Autodesk Inventor part; units mm, degrees
ref_plane "YZ Plane" through (0, 0, 0) normal (1, 0, 0) x (0, 1, 0)
ref_plane "XZ Plane" through (0, 0, 0) normal (0, 1, 0) x (-1, 0, 0)
ref_plane "XY Plane" through (0, 0, 0) normal (0, 0, 1) x (1, 0, 0)
sketch "Sketch1" plane through (0, 0, 0) normal (0, 1, 0) x (-1, 0, 0)
  line L0 (95, 92.5) -> (-95, 92.5)
  line L1 (-95, 92.5) -> (-95, -92.5)
  line L2 (-95, -92.5) -> (95, -92.5)
  line L3 (95, -92.5) -> (95, 92.5)
  point P0 (0, 0)
  dimension "d0" = 190
  dimension "d1" = 185
  dimension "d2" = 95
  dimension "d3" = 92.5
extrude "Extrusion1" add sketch "Sketch1" along normal blind 5
sketch "Sketch2" plane through (0, 0, 0) normal (0, -1, 0) x (1, 0, 0)
  line L0 (90, 87.5) -> (-90, 87.5)
  line L1 (-90, 87.5) -> (-90, -87.5)
  line L2 (-90, -87.5) -> (90, -87.5)
  line L3 (90, -87.5) -> (90, 87.5)
  line L4 (-95, 92.5) -> (95, 92.5)
  line L5 (-95, -92.5) -> (-95, 92.5)
  line L6 (95, -92.5) -> (-95, -92.5)
  line L7 (95, 92.5) -> (95, -92.5)
  line L8 (95, 92.5) -> (-95, 92.5)
  line L9 (-95, 92.5) -> (-95, -92.5)
  line L10 (-95, -92.5) -> (95, -92.5)
  line L11 (95, -92.5) -> (95, 92.5)
  point P0 (0, 0)
  dimension "d109" = 5
  dimension "d110" = 5
  dimension "d111" = 5
  dimension "d112" = 5
extrude "Extrusion2" add sketch "Sketch2" along normal blind 15
sketch "Sketch3" plane through (0, 5, 0) normal (0, 1, 0) x (1, 0, 0)
  circle A0 centre (-50, 0) radius 15.5
  point P0 (0, 0)
  dimension "d12" = 31
  dimension "d13" = 50
extrude "Extrusion3" cut sketch "Sketch3" against normal through all
sketch "Sketch4" plane through (0, 5, 0) normal (0, 1, 0) x (1, 0, 0)
  circle A0 centre (-50, 0) radius 15.5
  line L0 (-95, -92.5) -> (95, -92.5)
  line L1 (95, -92.5) -> (95, 92.5)
  line L2 (95, 92.5) -> (-95, 92.5)
  line L3 (-95, 92.5) -> (-95, -92.5)
  circle A1 centre (-77.5, -75) radius 7.5
  circle A2 centre (-77.5, 75) radius 7.5
  circle A3 centre (77.5, -75) radius 7.5
  circle A4 centre (77.5, 75) radius 7.5
  circle A5 centre (-77.5, -75) radius 8.5
  circle A6 centre (-77.5, 75) radius 8.5
  circle A7 centre (77.5, 75) radius 8.5
  circle A8 centre (77.5, -75) radius 8.5
  point P0 (0, 0)
  dimension "d16" = 15
  dimension "d17" = 17.5
  dimension "d18" = 17.5
  dimension "d19" = 15
  dimension "d20" = 15
  dimension "d21" = 15
  dimension "d22" = 17.5
  dimension "d23" = 17.5
  dimension "d24" = 17.5
  dimension "d25" = 17.5
  dimension "d26" = 17.5
  dimension "d27" = 17.5
  dimension "d28" = 17
  dimension "d29" = 17
  dimension "d30" = 17
  dimension "d31" = 17
  dimension "d34" = 75
  dimension "d35" = 77.5
extrude "Extrusion4" [suppressed]
sketch "Sketch8" plane through (0, 5, 0) normal (0, 1, 0) x (1, 0, 0)
  circle A0 centre (-50, 0) radius 15.5
  line L0 (-95, -92.5) -> (95, -92.5)
  line L1 (95, -92.5) -> (95, 92.5)
  line L2 (95, 92.5) -> (-95, 92.5)
  line L3 (-95, 92.5) -> (-95, -92.5)
  line L4 (-50, 13.5) -> (-50, -13.5)
  line L5 (-50, 13.5) -> (-95, 13.5)
  line L6 (-50, -13.5) -> (-95, -13.5)
  line L7 (-95, -13.5) -> (-95, 13.5)
  point P0 (0, 0)
  dimension "d51" = 27
  dimension "d52" = 13.5
  dimension "d62" = 31
extrude "Extrusion8" [suppressed]
sketch "Sketch10" plane through (-115, 5, -13.5) normal (0, 0, 1) x (1, 0, 0)
  line L0 (5, -20) -> (0, -20)
  line L1 (5, -5) -> (5, -20)
  line L2 (65, -5) -> (5, -5)
  line L3 (65, 0) -> (65, -5)
  line L4 (0, 0) -> (65, 0)
  line L5 (0, -20) -> (0, 0)
  line L6 (5, -17.5) -> (2.5, -17.5)
  line L7 (2.5, -17.5) -> (2.5, -2.5)
  line L8 (2.5, -2.5) -> (5, -2.5)
  line L9 (5, -2.5) -> (5, -17.5)
  line L10 (62.5, -5) -> (2.5, -5)
  line L11 (2.5, -5) -> (2.5, -2.5)
  line L12 (2.5, -2.5) -> (62.5, -2.5)
  line L13 (62.5, -2.5) -> (62.5, -5)
  point P0 (115, -5)
  dimension "d64" = 2.5
  dimension "d65" = 15
  dimension "d67" = 2.5
  dimension "d68" = 2.5
  dimension "d71" = 2.5
  dimension "d72" = 0
extrude "Extrusion10" [suppressed]
mirror "Mirror3" [suppressed]
sketch "Sketch12" plane through (0, 5, 0) normal (0, 1, 0) x (1, 0, 0)
  line L0 (-114.5, 13.5) -> (-109.5, 13.5)
  line L1 (-109.5, 13.5) -> (-109.5, 87.5)
  line L2 (-109.5, 87.5) -> (109.5, 87.5)
  line L3 (109.5, 87.5) -> (109.5, -87.5)
  line L4 (109.5, -87.5) -> (-109.5, -87.5)
  line L5 (-109.5, -87.5) -> (-109.5, -13.5)
  line L6 (-109.5, -13.5) -> (-114.5, -13.5)
  line L7 (-114.5, -13.5) -> (-114.5, -92.5)
  line L8 (-114.5, -92.5) -> (114.5, -92.5)
  line L9 (114.5, -92.5) -> (114.5, 92.5)
  line L10 (114.5, 92.5) -> (-114.5, 92.5)
  line L11 (-114.5, 92.5) -> (-114.5, 13.5)
  line L12 (-89.25, -92.5) -> (-79.25, -92.5)
  line L13 (-79.25, -92.5) -> (-79.25, -90)
  line L14 (-79.25, -90) -> (-89.25, -90)
  line L15 (-89.25, -90) -> (-89.25, -92.5)
  line L16 (79.25, -92.5) -> (89.25, -92.5)
  line L17 (89.25, -92.5) -> (89.25, -90)
  line L18 (89.25, -90) -> (79.25, -90)
  line L19 (79.25, -90) -> (79.25, -92.5)
  line L20 (-89.25, 92.5) -> (-79.25, 92.5)
  line L21 (-79.25, 92.5) -> (-79.25, 90)
  line L22 (-79.25, 90) -> (-89.25, 90)
  line L23 (-89.25, 90) -> (-89.25, 92.5)
  line L24 (79.25, 92.5) -> (89.25, 92.5)
  line L25 (89.25, 92.5) -> (89.25, 90)
  line L26 (89.25, 90) -> (79.25, 90)
  line L27 (79.25, 90) -> (79.25, 92.5)
  point P0 (0, 0)
  point P1 (0, 0)
  dimension "d87" = 10
  dimension "d88" = 2.5
  dimension "d89" = 20.25
  dimension "d90" = 10
  dimension "d91" = 2.5
  dimension "d92" = 20.25
  dimension "d93" = 2.5
  dimension "d94" = 10
  dimension "d95" = 20.25
  dimension "d96" = 2.5
  dimension "d97" = 10
  dimension "d98" = 20.25
  dimension "d113" = 5
  dimension "d114" = 5
  dimension "d115" = 5
  dimension "d116" = 5
  dimension "d117" = 5
  dimension "d118" = 229
  dimension "d119" = 229
  dimension "d120" = 158.5
  dimension "d121" = 79.25
  dimension "d122" = 79.25
extrude "Extrusion12" cut sketch "Sketch12" against normal blind 6 contours L10 L21 L22 L23 | L10 L25 L26 L27 | L8 L19 L18 L17 | L15 L14 L13 L8
sketch "Sketch13" plane through (0, -15, 0) normal (0, -1, 0) x (1, 0, 0)
  line L0 (-90, -87.5) -> (-90, 87.5)
  line L1 (-90, 87.5) -> (90, 87.5)
  line L2 (90, 87.5) -> (90, -87.5)
  line L3 (90, -87.5) -> (-90, -87.5)
  line L4 (-95, 92.5) -> (-95, -92.5)
  line L5 (-95, -92.5) -> (95, -92.5)
  line L6 (95, -92.5) -> (95, 92.5)
  line L7 (95, 92.5) -> (-95, 92.5)
  line L8 (112.75, -90.25) -> (-112.75, -90.25)
  line L9 (-112.75, -90.25) -> (-112.75, 90.25)
  line L10 (-112.75, 90.25) -> (112.75, 90.25)
  line L11 (112.75, 90.25) -> (112.75, -90.25)
  point P0 (0, 0)
  dimension "d101" = 185
  dimension "d102" = 180.5
  dimension "d104" = 225.5
  dimension "d105" = 112.75
  dimension "d106" = 90.25
extrude "Extrusion13" [suppressed]
equation "\"d110\" = d109"
equation "\"d111\" = d109"
equation "\"d112\" = d109"
equation "\"d18\" = d17"
equation "\"d19\" = d16"
equation "\"d20\" = d16"
equation "\"d21\" = d16"
equation "\"d22\" = d17"
equation "\"d23\" = d22"
equation "\"d24\" = d17"
equation "\"d25\" = d24"
equation "\"d26\" = d17"
equation "\"d27\" = d26"
equation "\"d29\" = d28"
equation "\"d30\" = d28"
equation "\"d31\" = d28"
equation "\"d52\" = 0.5 * d51"
equation "\"d90\" = d87"
equation "\"d91\" = d88"
equation "\"d92\" = d89"
equation "\"d93\" = d88"
equation "\"d94\" = d87"
equation "\"d95\" = d89"
equation "\"d96\" = d88"
equation "\"d97\" = d87"
equation "\"d98\" = d89"
properties part number "Bottom Roof"
Geometry: final body of the model. Coordinates: model frame, mm. A direction names the side the tool comes from. Coordinates: 2 decimals unless noted, no trailing zeros. Order: outer loops, then holes, each group sorted by start corner. A loop starts at its lowest first (then second) coordinate and runs counter-clockwise, first axis right, second up. Notation, with made-up numbers: M 76,74.5 L 131,74.5 A29 ccw 131,98.5 Z; hole C 30.25,44 d8. An arc over 180 degrees is marked long. One line per question, with ' | ' between items. Start each with the question number.
Item 1: Draft query along X for faces 1 (the flat face through (1, 5, 1)), 2 (the flat face through (90, -7, -1)), 3 (the flat face through (95, -5, 1)). Return one class per face: released by +X, released by -X, zero draft, split by the parting line, or undercut.
Item 2: Cut plane D-D, the plane z = -45. Return the cut outline in (x, y), then the cut area to 3 significant figures.
Item 3: Ray query, probe 1 along X at (y, z) = (1.55, 0); probe 2 along Z at (x, y) = (-54.5, -5); probe 3 along Z at (x, y) = (-50, 3.6). Return the intervals inside material, ascending. Write a range as [from, to].
Item 4: Pin query (flat end, axial travel): pin 1 Ø4 at (x, z) = (68.5, -6.5) entering from -Y; pin 2 Ø2 at (x, z) = (-86, 91.5) entering from +Y; pin 3 Ø1.8 at (x, y) = (-83, 0.5) entering from +Z. Return the tip coordinate at first contact, or that it passes through.
Item 5: Set-up query: faces 4 (the flat face through (84, 2, -90)), 5 (the flat face through (-1, -7, -87.5)), 6 (the flat face through (-84, 2, 90)). Return all of +Z, -Z, +X, -X, +Y, -Y with unobstructed straight access to the full face (end or side cutting, diameter ignored); none if empty.
Item 6: Cut plane C-C, the plane z = 0. Return the cut outline in (x, y), then the cut area to 3 significant figures.
Item 7: Cut plane A-A, the plane x = -50. Return the cut outline in (y, z).
Item 8: Cut plane B-B, the plane y = -9.25. Return the cut outline in (x, z), then the cut area to 3 significant figures.
A:
1) face 1: zero draft | face 2: undercut | face 3: released by +X
2) outline: M -95,-15 L -90,-15 L -90,0 L 90,0 L 90,-15 L 95,-15 L 95,5 L -95,5 Z | area: 1,100 mm2
3) probe 1: x = [-95, -65.5], [-34.5, 95] | probe 2: z = [-92.5, -87.5], [87.5, 92.5] | probe 3: z = [-92.5, -15.5], [15.5, 92.5]
4) pin 1: stops at y = 0 | pin 2: stops at y = -1 | pin 3: stops at z = 90
5) face 4: -Z, +Y | face 5: -Y | face 6: +Z, +Y
6) outline: M -95,-15 L -90,-15 L -90,0 L -65.5,0 L -65.5,5 L -95,5 Z; M -34.5,0 L 90,0 L 90,-15 L 95,-15 L 95,5 L -34.5,5 Z | area: 945 mm2
7) outline: M -15,-92.5 L 5,-92.5 L 5,-15.5 L 0,-15.5 L 0,-87.5 L -15,-87.5 Z; M -15,87.5 L 0,87.5 L 0,15.5 L 5,15.5 L 5,92.5 L -15,92.5 Z
8) outline: M -95,-92.5 L 95,-92.5 L 95,92.5 L -95,92.5 Z; hole M -90,-87.5 L 90,-87.5 L 90,87.5 L -90,87.5 Z | area: 3,650 mm2
